```python
from build123d import *

# Parameters (mm, degrees)
BOSS_EXTRU_1_DEPTH      = 10.16
ESQUISSE3_W             = 0.8
ESQUISSE3_H             = 1.27
ENL_V_MAT_EXTRU_1_DEPTH = 8.9
ESQUISSE4_W             = 2.4
ESQUISSE4_H             = 0.5
ENL_V_MAT_EXTRU_2_DEPTH = 11.16
ESQUISSE2_W             = 0.6
ESQUISSE2_H             = 0.6
BOSS_EXTRU_2_DEPTH      = 3.5
BOSS_EXTRU_2_DEPTH_BACK = 9
BOSS_EXTRU_3_DEPTH      = 7.62
CHANFREIN4_SIZE         = 0.15
CHANFREIN5_SIZE         = 0.4


with BuildPart() as part:
    # Esquisse1 → Boss.-Extru.1 (new body)
    with BuildSketch(Plane.XY):
        Polygon((0, 11.4), (0, 0), (5, 0), (5, 11.4), (4.2, 11.4), (4.2, 2.5), (0.8, 2.5), (0.8, 11.4), align=None)
    extrude(amount=BOSS_EXTRU_1_DEPTH)

    # Esquisse3 → Enlèv. mat.-Extru.1 (cut)
    with BuildSketch(Plane(origin=(0, 11.4, 0), x_dir=(1, 0, 0), z_dir=(0, 1, 0))):
        with Locations((0.4, -0.635)):
            Rectangle(ESQUISSE3_W, ESQUISSE3_H)
        with Locations((0.4, -9.525)):
            Rectangle(ESQUISSE3_W, ESQUISSE3_H)
    extrude(amount=-ENL_V_MAT_EXTRU_1_DEPTH, mode=Mode.SUBTRACT)

    # Esquisse4 → Enlèv. mat.-Extru.2 (cut, through all)
    with BuildSketch(Plane.XY.offset(10.16)):
        with Locations((2.5, 0.25)):
            Rectangle(ESQUISSE4_W, ESQUISSE4_H)
    extrude(amount=-ENL_V_MAT_EXTRU_2_DEPTH, mode=Mode.SUBTRACT)

    # Esquisse2 → Boss.-Extru.2 (add, two sides)
    with BuildSketch(Plane.XZ.offset(-0.5)) as boss_extru_2_sk:
        with Locations((2.5, 8.89)):
            Rectangle(ESQUISSE2_W, ESQUISSE2_H)
        with Locations((2.5, 1.27)):
            Rectangle(ESQUISSE2_W, ESQUISSE2_H)
        with Locations((2.5, 6.35)):
            Rectangle(ESQUISSE2_W, ESQUISSE2_H)
        with Locations((2.5, 3.81)):
            Rectangle(ESQUISSE2_W, ESQUISSE2_H)
    extrude(amount=BOSS_EXTRU_2_DEPTH)
    extrude(boss_extru_2_sk.sketch, amount=-BOSS_EXTRU_2_DEPTH_BACK)

    # Esquisse5 → Boss.-Extru.3 (add)
    with BuildSketch(Plane.XY.offset(8.89)):
        Polygon((0.8, 9.5), (1.2, 8.5), (0.8, 8.5), align=None)
    extrude(amount=-BOSS_EXTRU_3_DEPTH)

    # Chanfrein4
    chanfrein4_edges = [part.edges().sort_by_distance(p)[0] for p in [
        (2.8, 9.5, 6.35),
        (2.5, 9.5, 6.05),
        (2.2, 9.5, 6.35),
        (2.5, 9.5, 6.65),
        (2.8, -3, 6.35),
        (2.5, -3, 6.65),
        (2.2, -3, 6.35),
        (2.5, -3, 6.05),
        (2.8, 9.5, 3.81),
        (2.5, 9.5, 3.51),
        (2.2, 9.5, 3.81),
        (2.5, 9.5, 4.11),
        (2.8, -3, 3.81),
        (2.5, -3, 4.11),
        (2.2, -3, 3.81),
        (2.5, -3, 3.51),
        (2.8, 9.5, 8.89),
        (2.5, 9.5, 8.59),
        (2.2, 9.5, 8.89),
        (2.5, 9.5, 9.19),
        (2.8, -3, 8.89),
        (2.5, -3, 9.19),
        (2.2, -3, 8.89),
        (2.5, -3, 8.59),
        (2.8, 9.5, 1.27),
        (2.5, 9.5, 0.97),
        (2.2, 9.5, 1.27),
        (2.5, 9.5, 1.57),
        (2.8, -3, 1.27),
        (2.5, -3, 1.57),
        (2.2, -3, 1.27),
        (2.5, -3, 0.97),
    ]]
    chamfer(chanfrein4_edges, length=CHANFREIN4_SIZE)

    # Chanfrein5
    chanfrein5_edges = [part.edges().sort_by_distance(p)[0] for p in [
        (4.2, 11.4, 5.08),
        (0.8, 11.4, 5.08),
    ]]
    chamfer(chanfrein5_edges, length=CHANFREIN5_SIZE)


solid = part.part
```
Can you work these out from the model? Positions are in its coordinate system, mm. A direction names the side the tool comes from. Coordinates: 2 decimals unless noted, no trailing zeros. Loops run counter-clockwise (first coordinate to the right, second up) from the corner with the lowest first, then second, coordinate; pieces in that order, holes last. Notation, with made-up numbers: M 61.25,50.5 L 85.25,50.5 A21 cw 85.25,79.5 Z; hole C -13.75,-17.5 d5. An arc over 180 degrees is marked long. Put each result on its own line as item: value. Start each with the question number.
(1) Will these pins go through, and if not, where does the flat tip stop? pin 1 Ø1.5 at (x, z) = (3, 3.5) entering from +Y; pin 2 Ø0.5 at (y, z) = (-1, 1.5) entering from -X; pin 3 Ø0.5 at (x, y) = (2.5, 6) entering from -Z.
(2) Imagine slicing it at B-B on x = 0.6. List the corners of the cut face in (y, z) for me.
(3) Imagine slicing it at D-D on z = 7. List the corners of the cut face in (x, y) for me.
(4) I need wall thicknesses on probe 1 along X at (y, z) = (5.5, 6.5); probe 2 along Z at (x, y) = (2.4, 3); probe 3 along X at (y, z) = (8.25, 6). Which ranges of each line are inside material? Lowest first, please.
(5) Which directions (+Z, -Z, +X, -X, +Y, -Y) give clear straight access to the entire face, cutting with the end or side of a thin tool? Please do faces 1 (the face through (0.8, 10, 5)), 2 (the face through (1, 0, 5)), 3 (the face through (4, 0, 5)), 4 (the face through (0.5, 7, 8.89)), 5 (the face through (0.8, 5, 5)).
(6) We'd pull the mould along X, two halves only. Please class faces 6 (the face through (0, 6, 5)), 7 (the face through (2, 0.5, 5)), 8 (the face through (3, 2, 10.16)), 9 (the face through (5, 6, 5)): +X half, -X half, draft (parallel to the pull), parting line (faces both ways), or undercut.
(7) Imagine slicing it at A-A on y = 9.75. List the corners of the cut face in (x, z) for me.
(8) Imagine slicing it at C-C on y = 3.75. List the corners of the cut face in (x, z) for me, and give its area (3 significant figures).
Worked answers:
1. pin 1: stops at y = 9.5
1. pin 2: stops at x = 2.2
1. pin 3: stops at z = 0.97
2. outline: M 0,0 L 2.5,0 L 2.5,1.27 L 11.2,1.27 L 11.2,8.89 L 2.5,8.89 L 2.5,10.16 L 0,10.16 Z
3. outline: M 0,0 L 1.3,0 L 1.3,0.5 L 3.7,0.5 L 3.7,0 L 5,0 L 5,11.4 L 4.6,11.4 L 4.2,11 L 4.2,2.5 L 0.8,2.5 L 0.8,8.5 L 1.2,8.5 L 0.8,9.5 L 0.8,11 L 0.4,11.4 L 0,11.4 Z
4. probe 1: x = 0 to 0.8, 2.2 to 2.8, 4.2 to 5
4. probe 2: z = 0.97 to 1.57, 3.51 to 4.11, 6.05 to 6.65, 8.59 to 9.19
4. probe 3: x = 0 to 0.8, 4.2 to 5
5. face 1: +Z, -Z, +Y
5. face 2: +Z, -Z, -X, -Y
5. face 3: +Z, -Z, +X, -Y
5. face 4: +Z, -X, +Y
5. face 5: +Z, -Z
6. face 6: -X half
6. face 7: undercut
6. face 8: draft
6. face 9: +X half
7. outline: M 0,1.27 L 0.8,1.27 L 0.8,8.89 L 0,8.89 Z; M 4.2,0 L 5,0 L 5,10.16 L 4.2,10.16 Z
8. outline: M 0,1.27 L 0.8,1.27 L 0.8,8.89 L 0,8.89 Z; M 2.2,0.97 L 2.8,0.97 L 2.8,1.57 L 2.2,1.57 Z; M 2.2,3.51 L 2.8,3.51 L 2.8,4.11 L 2.2,4.11 Z; M 2.2,6.05 L 2.8,6.05 L 2.8,6.65 L 2.2,6.65 Z; M 2.2,8.59 L 2.8,8.59 L 2.8,9.19 L 2.2,9.19 Z; M 4.2,0 L 5,0 L 5,10.16 L 4.2,10.16 Z
8. area: 15.7 mm2
